```python
from build123d import *

# Parameters (mm, degrees)
SKETCH_1_W          = 15
SKETCH_1_H          = 10
SKETCH_1_W_2        = 12
SKETCH_1_H_2        = 8
EXTRUDE_1_DEPTH     = 70
SKETCH_2_R          = 1.6
CUT_EXTRUDE_1_DEPTH = 72.763500472
SKETCH_3_R          = 1.6
CUT_EXTRUDE_2_DEPTH = 72.107313267
SKETCH_4_R          = 1.6
CUT_EXTRUDE_3_DEPTH = 72.763500472


with BuildPart() as part:
    # ｽｹｯﾁ1 → ﾎﾞｽ - 押し出し1 (new body)
    with BuildSketch(Plane.XY):
        Rectangle(SKETCH_1_W, SKETCH_1_H)
        Rectangle(SKETCH_1_W_2, SKETCH_1_H_2, mode=Mode.SUBTRACT)
    extrude_1 = extrude(amount=EXTRUDE_1_DEPTH)

    # ｽｹｯﾁ2 → ｶｯﾄ - 押し出し1 (cut, through all)
    with BuildSketch(Plane(origin=(7.5, 0, 0), x_dir=(0, 0, -1), z_dir=(1, 0, 0))):
        with Locations((-13.5, 0)):
            Circle(SKETCH_2_R)
    cut_extrude_1 = extrude(amount=-CUT_EXTRUDE_1_DEPTH, mode=Mode.SUBTRACT)

    # ｽｹｯﾁ3 → ｶｯﾄ - 押し出し2 (cut, through all)
    with BuildSketch(Plane(origin=(0, 5, 0), x_dir=(1, 0, 0), z_dir=(0, 1, 0))):
        with Locations(Location((-2.5, -65, 0), (0, 0, 270))):
            Circle(SKETCH_3_R)
    cut_extrude_2 = extrude(amount=-CUT_EXTRUDE_2_DEPTH, mode=Mode.SUBTRACT)

    # ｽｹｯﾁ4 → ｶｯﾄ - 押し出し3 (cut, through all)
    with BuildSketch(Plane.ZY.offset(7.5)):
        with Locations((51.5, 0)):
            Circle(SKETCH_4_R)
    cut_extrude_3 = extrude(amount=-CUT_EXTRUDE_3_DEPTH, mode=Mode.SUBTRACT)

    # ﾐﾗｰ1: ﾎﾞｽ - 押し出し1, ｶｯﾄ - 押し出し1, ｶｯﾄ - 押し出し2, ｶｯﾄ - 押し出し3 across plane
    add(extrude_1.mirror(Plane(origin=(0, 0, 0), x_dir=(1, 0, 0), z_dir=(0, 0, -1))))
    add(cut_extrude_1.mirror(Plane(origin=(0, 0, 0), x_dir=(1, 0, 0), z_dir=(0, 0, -1))), mode=Mode.SUBTRACT)
    add(cut_extrude_2.mirror(Plane(origin=(0, 0, 0), x_dir=(1, 0, 0), z_dir=(0, 0, -1))), mode=Mode.SUBTRACT)
    add(cut_extrude_3.mirror(Plane(origin=(0, 0, 0), x_dir=(1, 0, 0), z_dir=(0, 0, -1))), mode=Mode.SUBTRACT)


solid = part.part
```
Check sheet for the modelled part. Datum: model origin and axes. Units: mm. A direction names the side the tool comes from. Round coordinates to 2 decimals unless told otherwise and drop trailing zeros. Order: outer loops, then holes, each group sorted by start corner. A loop starts at its lowest first (then second) coordinate and runs counter-clockwise, first axis right, second up. Notation, with made-up numbers: M 79,72 L 103,72 A28 cw 103,111 Z; hole C 29.5,88 d9. An arc over 180 degrees is marked long. Answer in a Markdown table with one row per item.
(1) Draft check along X on faces 1 (the flat face through (6, 0, 1)), 2 (the cylindrical face through (6.76, 0.07, -15.1)), 3 (the flat face through (-7.5, 0, 1)). Enter one of: +X half, -X half, draft (parallel to the pull), parting line (faces both ways), or undercut.
Findings:
| item | result |
|---|---|
| face 1 | undercut |
| face 2 | draft |
| face 3 | -X half |
(2) Gauge pin test, flat end, axial feed: pin 1 (2.5 mm diameter, centred on y = 0, z = 51.5, fed in from -X). Record the tip position at first contact, or that the pin passes through.
Findings:
| item | result |
|---|---|
| pin 1 | passes through |
(3) Section check B-B on z = -51.5. Record the boundary of the cut face in (x, y).
Findings:
| item | result |
|---|---|
| outline | M -7.5,-5 L 7.5,-5 L 7.5,-1.6 L 6,-1.6 L 6,-4 L -6,-4 L -6,-1.6 L -7.5,-1.6 Z; M -7.5,1.6 L -6,1.6 L -6,4 L 6,4 L 6,1.6 L 7.5,1.6 L 7.5,5 L -7.5,5 Z |
(4) Section check D-D on z = 39. Record the boundary of the cut face in (x, y).
Findings:
| item | result |
|---|---|
| outline | M -7.5,-5 L 7.5,-5 L 7.5,5 L -7.5,5 Z; hole M -6,-4 L 6,-4 L 6,4 L -6,4 Z |
(5) Set-up check for faces 4 (the flat face through (0, 4, 1)), 5 (the cylindrical face through (6.74, 0.481, -53.026)): record each of +Z, -Z, +X, -X, +Y, -Y from which the full face is reachable in a straight line by a thin tool's end or side.
Findings:
| item | result |
|---|---|
| face 4 | +Z, -Z |
| face 5 | +X, -X |
(6) Section check A-A on x = -2.5. Record the boundary of the cut face in (y, z).
Findings:
| item | result |
|---|---|
| outline | M -5,-70 L -4,-70 L -4,-66.6 L -5,-66.6 Z; M -5,-63.4 L -4,-63.4 L -4,63.4 L -5,63.4 Z; M -5,66.6 L -4,66.6 L -4,70 L -5,70 Z; M 4,-70 L 5,-70 L 5,-66.6 L 4,-66.6 Z; M 4,-63.4 L 5,-63.4 L 5,63.4 L 4,63.4 Z; M 4,66.6 L 5,66.6 L 5,70 L 4,70 Z |
(7) Material ranges on line 1 along X through (y, z) = (-2.25, -14.5); line 2 along Y through (x, z) = (-0.5, 28); line 3 along Y through (x, z) = (-6.5, 51.5), recorded low to high. Write a range as from..to.
Findings:
| item | result |
|---|---|
| line 1 | x = -7.5..-6, 6..7.5 |
| line 2 | y = -5..-4, 4..5 |
| line 3 | y = -5..-1.6, 1.6..5 |
(8) Section check C-C on x = 3. Record the boundary of the cut face in (y, z).
Findings:
| item | result |
|---|---|
| outline | M -5,-70 L -4,-70 L -4,70 L -5,70 Z; M 4,-70 L 5,-70 L 5,70 L 4,70 Z |
